Check sheet for the modelled part. Datum: model origin and axes. Units: mm. A direction names the side the tool comes from. Round coordinates to 2 decimals unless told otherwise and drop trailing zeros. Write each loop counter-clockwise with the first axis right and the second up, starting at its lowest first coordinate (ties: lowest second). Pieces come first, ordered by that corner, then holes. Notation, with made-up numbers: (66, 42.5) -> (86, 42.5) arc R23 cw to (86, 60.5) -> close; hole circle Ø6 at (-14, -26). An arc over 180 degrees is marked (long way). One line per item, written item: value.
Autodesk Inventor part; units mm, degrees
ref_plane "YZ Plane" through (0, 0, 0) normal (1, 0, 0) x (0, 1, 0)
ref_plane "XZ Plane" through (0, 0, 0) normal (0, 1, 0) x (-1, 0, 0)
ref_plane "XY Plane" through (0, 0, 0) normal (0, 0, 1) x (1, 0, 0)
sketch "Sketch1" plane through (0, 0, 0) normal (1, 0, 0) x (0, 1, 0)
  line L0 (0, 0) -> (0, -9.85)
  line L1 (0, -9.85) -> (-120, -9.85)
  line L2 (-120, -9.85) -> (-120, -37.5)
  line L3 (-120, -37.5) -> (-135, -37.5)
  line L4 (-135, -37.5) -> (-135, 0)
  line L5 (-135, 0) -> (0, 0)
  line L6 (-135, 0) -> (-135, 22.5)
  line L7 (-135, 22.5) -> (-150, 22.5)
  line L8 (-135, 0) -> (-135, -22.5)
  line L9 (-135, -22.5) -> (-150, -22.5)
  arc A0 (-150, 22.5) -> (-181.8198, 0) centre (-150, -11.25) ccw
  arc A1 (-181.8198, 0) -> (-150, -22.5) centre (-150, 11.25) ccw
  arc A2 (-120, -10.1) -> (-119.8236, -9.85) centre (-150, 11.25) ccw
  circle A3 centre (-160, 0) radius 10
  dimension "d0" = 9.85
  dimension "d1" = 120
  dimension "d2" = 27.65
  dimension "d3" = 15
  dimension "d4" = 22.5
  dimension "d5" = 15
  dimension "d6" = 22.5
  dimension "d14" = 33.75
  dimension "d15" = 33.75
  dimension "d16" = 20
  dimension "d17" = 25
revolve "Revolution1" add sketch "Sketch1" angle 360 about axis through (0, -135, 0) along (0, 1, 0) contours L0 L1 L2 L3 L4 L5
extrude "Extrusion1" add sketch "Sketch1" along normal mid plane 15 contours L4 L9 A1 A0 L7 L6
fillet "Fillet1" radius 4 7 edges at (0, -120, 37.5) (0, -135, 37.5) (0, -120, 9.85) (7.5, -135, 0) (0, -135, 22.5) (0, -135, -22.5) (-7.5, -135, 0)
fillet "Fillet2" radius 4 1 edges at (0, -181.8198, 0)
properties material "Aluminum 6061"
Item 1: Sectioned sample at B-B (y = -35). Enter the section's corners in (x, z).
Result set:
outline: circle Ø19.7 at (0, 0)
Item 2: Release check for a two-part mould opening along Z. For faces 4 (the flat face through (0, -144, 22.5)), 5 (the flat face through (0, 0, 0)), 6 (the cylindrical face through (-0.105, -150.763, 3.83)), 7 (the flat face through (0, -144, -22.5)) record: pulls with the +Z half, pulls with the -Z half, needs draft (parallel to the pull), parting line crosses it, or undercut.
Result set:
face 4: pulls with the +Z half
face 5: needs draft
face 6: undercut
face 7: pulls with the -Z half
Item 3: Depth check by flat-ended pin: pin 1 (5 mm diameter, centred on y = -133, z = -7, fed in from -X); pin 2 (6 mm diameter, centred on x = 27, y = -123.5, fed in from -Z); pin 3 (2 mm diameter, centred on y = -150, z = -7.5, fed in from -X); pin 4 (8 mm diameter, centred on x = 12, y = -148, fed in from +Z). Enter the tip coordinate at first touch or a pass-through.
Result set:
pin 1: x = -37.13
pin 2: z = -28.8
pin 3: x = -7.5
pin 4: through
Item 4: Sectioned sample at A-A (y = -160). Enter the section's corners in (x, z).
Result set:
outline: (-7.5, -20.98) -> (7.5, -20.98) -> (7.5, -10) -> (-7.5, -10) -> close; (-7.5, 10) -> (7.5, 10) -> (7.5, 20.98) -> (-7.5, 20.98) -> close
Item 5: Material ranges on line 1 along Y through (x, z) = (14, 16); line 2 along Z through (x, y) = (-1, -160); line 3 along X through (y, z) = (-147.5, 14), recorded low to high.
Result set:
line 1: -135 to -120
line 2: -20.98 to -10, 10 to 20.98
line 3: -7.5 to 7.5
Item 6: Tool access check on faces 1 (the flat face through (7.5, -151, 5)), 2 (the cylindrical face through (-5.99, -58.81, 7.82)), 3 (the flat face through (-7.5, -151, 5)). Record the directions out of +Z, -Z, +X, -X, +Y, -Y that give a thin tool (end or side, any length) a straight path to the whole face; none if there is none.
Result set:
face 1: +Z, -Z, +X, -Y
face 2: +Y
face 3: +Z, -Z, -X, -Y
